```python
from build123d import *

# Parameters (mm, degrees)
SKETCH1_W           = 44.45
SKETCH1_H           = 6.35
BOSS_EXTRUDE1_DEPTH = 76.2
SKETCH2_W           = 38.1
SKETCH2_H           = 3.175
CUT_EXTRUDE1_DEPTH  = 73.025
SKETCH4_R           = 1.25
CUT_EXTRUDE2_DEPTH  = 4.175


with BuildPart() as part:
    # Sketch1 → Boss-Extrude1 (new body)
    with BuildSketch(Plane(origin=(0, 0, 0), x_dir=(1, 0, 0), z_dir=(0, 1, 0))):
        Rectangle(SKETCH1_W, SKETCH1_H)
    extrude(amount=BOSS_EXTRUDE1_DEPTH)

    # Sketch2 → Cut-Extrude1 (cut)
    with BuildSketch(Plane(origin=(0, 76.2, 0), x_dir=(1, 0, 0), z_dir=(0, 1, 0))):
        with Locations((0, 1.5875)):
            Rectangle(SKETCH2_W, SKETCH2_H)
    extrude(amount=-CUT_EXTRUDE1_DEPTH, mode=Mode.SUBTRACT)

    # Sketch4 → Cut-Extrude2 (cut, through all)
    with BuildSketch(Plane(origin=(0, 0, 0), x_dir=(-1, 0, 0), z_dir=(0, 0, -1))):
        with Locations((-9.525, 66.675)):
            Circle(SKETCH4_R)
        with Locations((9.525, 66.675)):
            Circle(SKETCH4_R)
        with Locations((-15.875, 15.875)):
            Circle(SKETCH4_R)
        with Locations((15.875, 15.875)):
            Circle(SKETCH4_R)
    extrude(amount=-CUT_EXTRUDE2_DEPTH, mode=Mode.SUBTRACT)


solid = part.part
```
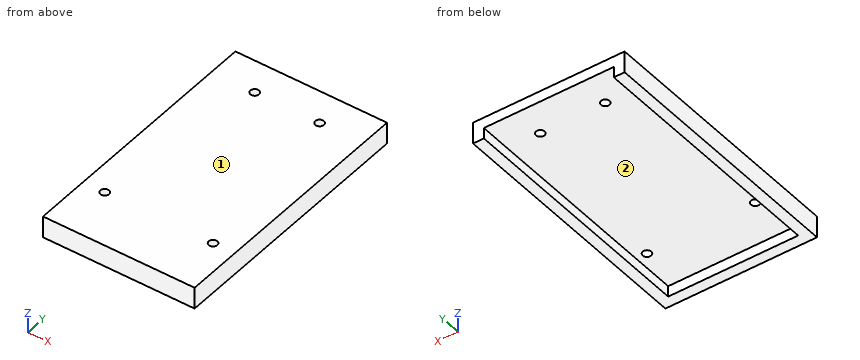
Input: part model. Units: mm. Frame: model coordinates. Face numbers are marked on the shaded views. A direction names the side the tool comes from. Round coordinates to 2 decimals unless told otherwise and drop trailing zeros. Write each loop counter-clockwise with the first axis right and the second up, starting at its lowest first coordinate (ties: lowest second). Pieces come first, ordered by that corner, then holes. Notation, with made-up numbers: (64.5, -12) - (122.5, -12) arc R21 ccw to (122.5, 10) - close; hole circle Ø8 at (-5, -17). An arc over 180 degrees is marked (long way). Write item = value, one per line.
(1) Section query A-A on z = -2. Output: boundary loops of the cut face in (x, y) (3 decimals).
Geometry check:
outline = (-22.225, 0) - (22.225, 0) - (22.225, 76.2) - (19.05, 76.2) - (19.05, 3.175) - (-19.05, 3.175) - (-19.05, 76.2) - (-22.225, 76.2) - close
(2) Section query C-C on x = 2.5. Output: boundary loops of the cut face in (y, z) (3 decimals), then the cut area to 3 significant figures.
Geometry check:
outline = (0, -3.175) - (3.175, -3.175) - (3.175, 0) - (76.2, 0) - (76.2, 3.175) - (0, 3.175) - close
area = 252 mm^2
(3) Section query B-B on y = 8. Output: boundary loops of the cut face in (x, z) (3 decimals), then the cut area to 3 significant figures.
Geometry check:
outline = (-22.225, -3.175) - (-19.05, -3.175) - (-19.05, 0) - (19.05, 0) - (19.05, -3.175) - (22.225, -3.175) - (22.225, 3.175) - (-22.225, 3.175) - close
area = 161 mm^2
(4) Contact query for flat-ended pins moving along their axis: pin 1 Ø19 at (x, y) = (-3, 32) entering from -Z; pin 2 Ø2.5 at (x, z) = (-8, -2) entering from +Y (3 decimals). Output: stop coordinate, or through.
Geometry check:
pin_1 = 0
pin_2 = 3.175
(5) Material intervals for probe 1 along X at (y, z) = (16, 2) (3 decimals); probe 2 along X at (y, z) = (15, -1.5) (3 decimals); probe 3 along Y at (x, z) = (-16, 2.25), sorted ascending.
Geometry check:
probe_1 = -22.225 to -17.119, -14.631 to 14.631, 17.119 to 22.225
probe_2 = -22.225 to -19.05, 19.05 to 22.225
probe_3 = 0 to 14.63, 17.12 to 76.2
(6) Access query for the marked faces 1 and 2. Directions: +Z, -Z, +X, -X, +Y, -Y. A direction counts if a zero-diameter tool reaches every point of the face in a straight line with its end or side. Return the directions, or none.
Geometry check:
face_1 = +Z, +X, -X, +Y, -Y
face_2 = -Z, +Y
